Autodesk Inventor part; units mm, degrees
ref_plane "YZ Plane" through (0, 0, 0) normal (1, 0, 0) x (0, 1, 0)
ref_plane "XZ Plane" through (0, 0, 0) normal (0, 1, 0) x (-1, 0, 0)
ref_plane "XY Plane" through (0, 0, 0) normal (0, 0, 1) x (1, 0, 0)
sketch "Sketch1" plane through (0, 0, 0) normal (0, 0, 1) x (1, 0, 0)
  line L0 (12.7, -25.4) -> (-12.7, -25.4)
  line L1 (-12.7, -25.4) -> (-12.7, 25.4)
  line L2 (-12.7, 25.4) -> (12.7, 25.4)
  line L3 (12.7, 25.4) -> (12.7, -25.4)
  line L4 (12.7, -25.4) -> (-12.7, 25.4) construction
  line L5 (-12.7, -25.4) -> (12.7, 25.4) construction
  line L6 (10.16, -22.86) -> (-10.16, -22.86)
  line L7 (-10.16, -22.86) -> (-10.16, 22.86)
  line L8 (-10.16, 22.86) -> (10.16, 22.86)
  line L9 (10.16, 22.86) -> (10.16, -22.86)
  line L10 (10.16, -22.86) -> (-10.16, 22.86) construction
  line L11 (-10.16, -22.86) -> (10.16, 22.86) construction
  point P0 (0, 0)
  dimension "d0" = 25.4
  dimension "d1" = 50.8
  dimension "d2" = 20.32
  dimension "d3" = 45.72
extrude "Extrusion1" add sketch "Sketch1" along normal mid plane 254
sketch "Sketch2" plane through (-12.7, 25.4, 127) normal (0, 1, 0) x (1, 0, 0)
  line L0 (0, 0) -> (0, 254)
  line L1 (25.4, 0) -> (0, 0)
  point P0 (12.7, 127)
  point P1 (12.7, 12.7)
  dimension "d6" = 12.7
  dimension "d7" = 12.7
hole "Hole1" at (0, 25.4, 114.3) direction (0, -1, 0) diameter 4.1402 end through all
pattern_linear "Rectangular Pattern1" count 10 spacing 25.4 along (0, 0, -1) of "Hole1"
properties part number "Intake_vertical"
Source: CAD feature listing. Evaluate the final solid. Frame: model axes, mm. A direction names the side the tool comes from. Round coordinates to 2 decimals unless told otherwise and drop trailing zeros. Loops run counter-clockwise (first coordinate to the right, second up) from the corner with the lowest first, then second, coordinate; pieces in that order, holes last. Notation, with made-up numbers: (-15.75, -37) - (16.25, -37) arc R16 cw to (16.25, -13) - close; hole circle Ø10 at (-36.5, 4.5). An arc over 180 degrees is marked (long way). Write item = value, one per line. Start each with the question number.
(1) Pull-direction query (X, two-part tool) for faces 1 (the face through (-0.09, 24.11, -90.97)), 2 (the face through (0, 25.4, -2)), 3 (the face through (-12.7, 0, -2)); classes: +X half, -X half, draft (parallel to the pull), parting line (faces both ways), or undercut.
(2) Ray query, line 1 along X through (y, z) = (-20.5, -78); line 2 along Y through (x, z) = (4.25, -83); line 3 along X through (y, z) = (23.9, 63.5). Return the intervals inside material, ascending. Write a range as from..to.
(3) Section query B-B, the plane y = -7. Output: boundary loops of the cut face in (x, z), plus the area to 3 significant figures.
(4) Section query C-C, the plane z = -0.5. Output: boundary loops of the cut face in (x, y).
(5) Set-up query: faces 4 (the face through (-0.09, 24.11, 36.03)), 5 (the face through (10.16, 0, -2)). Return all of +Z, -Z, +X, -X, +Y, -Y with unobstructed straight access to the full face (end or side cutting, diameter ignored); none if empty.
(6) Pin query (flat end, axial travel): pin 1 (10 mm diameter, centred on x = -5, y = 19, fed in from -Z). Return the tip coordinate at first contact, or that it passes through.
(7) Section query A-A, the plane x = -6.75. Output: boundary loops of the cut face in (y, z), plus the area to 3 significant figures.
Conclusion:
q1.face_1 = undercut
q1.face_2 = draft
q1.face_3 = -X half
q2.line_1 = -12.7..-10.16, 10.16..12.7
q2.line_2 = -25.4..-22.86, 22.86..25.4
q2.line_3 = -12.7..-2.07, 2.07..12.7
q3.outline = (-12.7, -127) - (-10.16, -127) - (-10.16, 127) - (-12.7, 127) - close; (10.16, -127) - (12.7, -127) - (12.7, 127) - (10.16, 127) - close
q3.area = 1,290 mm2
q4.outline = (-12.7, -25.4) - (12.7, -25.4) - (12.7, 25.4) - (-12.7, 25.4) - close; hole (-10.16, -22.86) - (10.16, -22.86) - (10.16, 22.86) - (-10.16, 22.86) - close
q5.face_4 = +Y, -Y
q5.face_5 = +Z, -Z
q6.pin_1 = -127
q7.outline = (-25.4, -127) - (-22.86, -127) - (-22.86, 127) - (-25.4, 127) - close; (22.86, -127) - (25.4, -127) - (25.4, 127) - (22.86, 127) - close
q7.area = 1,290 mm2
